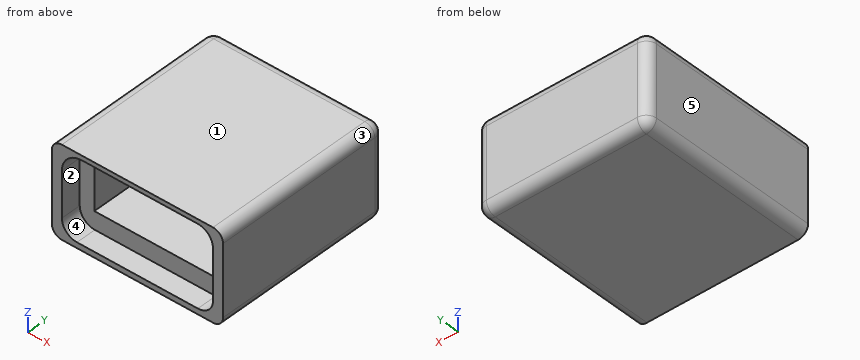
```python
from build123d import *

# Parameters (mm, degrees)
F1_DEPTH = 18
F2_W     = 12.1
F2_H     = 4.5
F3_DEPTH = 14.43852
F5_DEPTH = 2
F6_R     = 1


# Not quite as in the source:
# - a feature names something its author has since deleted; it is built from what else it names


with BuildPart() as f1:
    # F0 (on Front) → F1 (new body)
    with BuildSketch(Plane.XZ):
        with BuildLine():
            ThreePointArc((8.5, 3.4460804202), (8.2071067812, 4.1531872014), (7.5, 4.4460804202))
            Line((7.5, 4.4460804202), (-7.5, 4.4460804202))
            ThreePointArc((-7.5, 4.4460804202), (-8.2071067812, 4.1531872014), (-8.5, 3.4460804202))
            Line((-8.5, 3.4460804202), (-8.5, -3.5539195798))
            ThreePointArc((-8.5, -3.5539195798), (-8.2071067812, -4.261026361), (-7.5, -4.5539195798))
            Line((-7.5, -4.5539195798), (7.5, -4.5539195798))
            ThreePointArc((7.5, -4.5539195798), (8.2071067812, -4.261026361), (8.5, -3.5539195798))
            Line((8.5, -3.5539195798), (8.5, 3.4460804202))
        make_face()
    extrude(amount=-F1_DEPTH)

    # F2 (on face) → F3 (cut)
    with BuildSketch(Plane.XZ):
        Rectangle(F2_W, F2_H)
    extrude(amount=-F3_DEPTH, mode=Mode.SUBTRACT)

    # F4 (on face) → F5 (cut)
    with BuildSketch(Plane.XZ):
        with BuildLine():
            Line((-6, -4), (6, -4))
            ThreePointArc((6, -4), (7.0606601718, -3.5606601718), (7.5, -2.5))
            Line((7.5, -2.5), (7.5, 2.5))
            ThreePointArc((7.5, 2.5), (7.0606601718, 3.5606601718), (6, 4))
            Line((6, 4), (-5.5, 4))
            ThreePointArc((-5.5, 4), (-6.9142135624, 3.4142135624), (-7.5, 2))
            Line((-7.5, 2), (-7.5, -2.5))
            ThreePointArc((-7.5, -2.5), (-7.0606601718, -3.5606601718), (-6, -4))
        make_face()
    extrude(amount=-F5_DEPTH, mode=Mode.SUBTRACT)

    # F6
    f6_edges = [f1.edges().sort_by_distance(p)[0] for p in [
        (8.207107, 18, -4.261026),
        (8.5, 18, -0.05392),
        (8.207107, 18, 4.153187),
        (0, 18, 4.44608),
        (-8.207107, 18, 4.153187),
        (-8.5, 18, -0.05392),
        (-8.207107, 18, -4.261026),
        (0, 18, -4.55392),
    ]]
    fillet(f6_edges, radius=F6_R)


solid = f1.part
```
Check sheet for the modelled part. Datum: model origin and axes. Units: mm. Face numbers are marked on the shaded views. A direction names the side the tool comes from. Round coordinates to 2 decimals unless told otherwise and drop trailing zeros. Order: outer loops, then holes, each group sorted by start corner. A loop starts at its lowest first (then second) coordinate and runs counter-clockwise, first axis right, second up. Notation, with made-up numbers: (57.25, 66.5) -> (95.25, 66.5) arc R30 cw to (95.25, 92.5) -> close; hole circle Ø6 at (36, 81). An arc over 180 degrees is marked (long way). Use CSV: the item, a comma, the result in double quotes.
(1) Tool access check on the marked faces 4 and 5. Record the directions out of +Z, -Z, +X, -X, +Y, -Y that give a thin tool (end or side, any length) a straight path to the whole face; none if there is none.
Worked out:
face 4,"-Y"
face 5,"+Z, -Z, -X, +Y, -Y"
(2) Cross-section at C-C (x = 0.75). Record the boundary of the cut face in (y, z).
Worked out:
outline,"(0, -4.55) -> (17, -4.55) arc R1 ccw to (18, -3.55) -> (18, 3.45) arc R1 ccw to (17, 4.45) -> (0, 4.45) -> (0, 4) -> (2, 4) -> (2, 2.25) -> (14.44, 2.25) -> (14.44, -2.25) -> (2, -2.25) -> (2, -4) -> (0, -4) -> close"
(3) Material ranges on line 1 along Z through (x, y) = (-2.25, 12); line 2 along X through (y, z) = (5.75, 2); line 3 along Z through (x, y) = (-0.25, 1.5), recorded low to high. Write a range as from..to.
Worked out:
line 1,"-4.55..-2.25, 2.25..4.45"
line 2,"-8.5..-6.05, 6.05..8.5"
line 3,"-4.55..-4, 4..4.45"
(4) Draft check along X on the marked faces 1, 2 and 3. Enter one of: pulls with the +X half, pulls with the -X half, needs draft (parallel to the pull), parting line crosses it, or undercut.
Worked out:
face 1,"needs draft"
face 2,"undercut"
face 3,"pulls with the +X half"
(5) Cross-section at A-A (y = 8). Record the boundary of the cut face in (x, z), and give its area (3 significant figures).
Worked out:
outline,"(-8.5, -3.55) arc R1 ccw to (-7.5, -4.55) -> (7.5, -4.55) arc R1 ccw to (8.5, -3.55) -> (8.5, 3.45) arc R1 ccw to (7.5, 4.45) -> (-7.5, 4.45) arc R1 ccw to (-8.5, 3.45) -> close; hole (-6.05, -2.25) -> (6.05, -2.25) -> (6.05, 2.25) -> (-6.05, 2.25) -> close"
area,"97.7 mm²"
(6) Depth check by flat-ended pin: pin 1 (1.3 mm diameter, centred on x = 0, z = -0.5, fed in from -Y). Enter the tip coordinate at first touch or a pass-through.
Worked out:
pin 1,"y = 14.44"
(7) Cross-section at B-B (z = 0). Record the boundary of the cut face in (x, y).
Worked out:
outline,"(-8.5, 0) -> (-7.5, 0) -> (-7.5, 2) -> (-6.05, 2) -> (-6.05, 14.44) -> (6.05, 14.44) -> (6.05, 2) -> (7.5, 2) -> (7.5, 0) -> (8.5, 0) -> (8.5, 17) arc R1 ccw to (7.5, 18) -> (-7.5, 18) arc R1 ccw to (-8.5, 17) -> close"
(8) Cross-section at D-D (z = -3). Record the boundary of the cut face in (x, y), and give its area (3 significant figures).
Worked out:
outline,"(-8.5, 0) -> (-7.41, 0) -> (-7.41, 2) -> (7.41, 2) -> (7.41, 0) -> (8.5, 0) -> (8.5, 17) arc R1 ccw to (7.5, 18) -> (-7.5, 18) arc R1 ccw to (-8.5, 17) -> close"
area,"276 mm²"
